Here's how the part is built. I have some questions about the finished solid (model axes, mm). Round coordinates to 2 decimals unless told otherwise and drop trailing zeros. Write each loop counter-clockwise with the first axis right and the second up, starting at its lowest first coordinate (ties: lowest second). Pieces come first, ordered by that corner, then holes. Notation, with made-up numbers: M 20,59 L 41,59 A15 cw 41,88 Z; hole C 55.5,-23 d4. An arc over 180 degrees is marked long. Use one line per item in the form item = value. Start each with the question number.
Q1. I'm going to push a flat-ended pin straight in: pin 1 Ø2.5 at (x, z) = (15.98, -0.88) entering from +Y. Where does the tip first touch, or does it pass through?
Q2. I want a section at B-B on x = 0.5. List the corners of the cut face in (y, z) for me (3 decimals).
Q3. I want a section at D-D on y = 1.5. List the corners of the cut face in (x, z) for me (3 decimals), and give its area (3 significant figures).
Q4. I want a section at A-A on z = 3.5. List the corners of the cut face in (x, y) for me.
Q5. I need wall thicknesses on line 1 along X through (y, z) = (1.75, -2); line 2 along X through (y, z) = (4.75, -0.25); line 3 along X through (y, z) = (3.75, 4). Which ranges of each line are inside material? Lowest first, please. Write a range as from..to.
Q6. We'd pull the mould along Z, two halves only. Please class faces 1 (the face through (20, 5, 0)), 2 (the face through (0, 9, 4.875)), 3 (the face through (-14.49, 5.42, -1.07)): +Z half, -Z half, draft (parallel to the pull), parting line (faces both ways), or undercut.
Q7. I want a section at C-C on z = -0.5. List the corners of the cut face in (x, y) for me.
```python
from build123d import *

# Parameters (mm, degrees)
SKETCH1_W           = 40
SKETCH1_H           = 9.75
SKETCH1_R           = 1.5
BOSS_EXTRUDE1_DEPTH = 11
CUT_EXTRUDE1_REACH  = 26.821


with BuildPart() as part:
    # Sketch1 → Boss-Extrude1 (new body)
    with BuildSketch(Plane(origin=(0, 0, 0), x_dir=(1, 0, 0), z_dir=(0, 1, 0))):
        Rectangle(SKETCH1_W, SKETCH1_H)
        with Locations(Location((-15.976056303, 0.875, 0), (0, 0, 270))):
            Circle(SKETCH1_R, mode=Mode.SUBTRACT)
        with Locations(Location((15.976056303, 0.875, 0), (0, 0, 90))):
            Circle(SKETCH1_R, mode=Mode.SUBTRACT)
    extrude(amount=BOSS_EXTRUDE1_DEPTH)

    # Sketch2 → Cut-Extrude1 (cut, up to next)
    with BuildSketch(Plane.XY.offset(4.875), mode=Mode.PRIVATE) as cut_extrude1_sk1:
        with BuildLine():
            ThreePointArc((3, 5.5), (2.121320344, 7.621320344), (0, 8.5))
            Line((0, 8.5), (0, 2.5))
            ThreePointArc((0, 2.5), (2.121320344, 3.378679656), (3, 5.5))
        make_face()
    cut_extrude1_tool1 = extrude(cut_extrude1_sk1.sketch, amount=-CUT_EXTRUDE1_REACH, mode=Mode.PRIVATE) & part.part
    # Sketch2 → Cut-Extrude1 (cut, up to next)
    with BuildSketch(Plane.XY.offset(4.875), mode=Mode.PRIVATE) as cut_extrude1_sk2:
        with BuildLine():
            Line((0, 2.5), (0, 8.5))
            ThreePointArc((0, 8.5), (-3, 5.5), (0, 2.5))
        make_face()
    cut_extrude1_tool2 = extrude(cut_extrude1_sk2.sketch, amount=-CUT_EXTRUDE1_REACH, mode=Mode.PRIVATE) & part.part
    # Sketch2 → Cut-Extrude1 (cut, up to next)
    with BuildSketch(Plane.XY.offset(4.875), mode=Mode.PRIVATE) as cut_extrude1_sk3:
        with BuildLine():
            ThreePointArc((3, 5.5), (2.121320344, 7.621320344), (0, 8.5))
            Line((0, 8.5), (0, 2.5))
            ThreePointArc((0, 2.5), (2.121320344, 3.378679656), (3, 5.5))
        make_face()
    cut_extrude1_tool3 = extrude(cut_extrude1_sk3.sketch, amount=-CUT_EXTRUDE1_REACH, mode=Mode.PRIVATE) & part.part
    # Sketch2 → Cut-Extrude1 (cut, up to next)
    with BuildSketch(Plane.XY.offset(4.875), mode=Mode.PRIVATE) as cut_extrude1_sk4:
        with BuildLine():
            Line((0, 2.5), (0, 8.5))
            ThreePointArc((0, 8.5), (-3, 5.5), (0, 2.5))
        make_face()
    cut_extrude1_tool4 = extrude(cut_extrude1_sk4.sketch, amount=-CUT_EXTRUDE1_REACH, mode=Mode.PRIVATE) & part.part
    add(cut_extrude1_tool1.solids().sort_by_distance((1.27324, 5.5, 4.875))[0], mode=Mode.SUBTRACT)
    add(cut_extrude1_tool2.solids().sort_by_distance((-1.27324, 5.5, 4.875))[0], mode=Mode.SUBTRACT)
    add(cut_extrude1_tool3.solids().sort_by_distance((1.27324, 5.5, 4.875))[0], mode=Mode.SUBTRACT)
    add(cut_extrude1_tool4.solids().sort_by_distance((-1.27324, 5.5, 4.875))[0], mode=Mode.SUBTRACT)


solid = part.part
```
Reported:
q1.pin_1 = through
q2.outline = M 0,-4.875 L 2.542,-4.875 L 2.542,4.875 L 0,4.875 Z; M 8.458,-4.875 L 11,-4.875 L 11,4.875 L 8.458,4.875 Z
q3.outline = M -20,-4.875 L 20,-4.875 L 20,4.875 L -20,4.875 Z; hole C -15.976,-0.875 d3; hole C 15.976,-0.875 d3
q3.area = 376 mm^2
q4.outline = M -20,0 L 20,0 L 20,11 L -20,11 Z; hole C 0,5.5 d6
q5.line_1 = -20..-16.97, -14.98..14.98, 16.97..20
q5.line_2 = -20..-17.34, -14.61..-2.9, 2.9..14.61, 17.34..20
q5.line_3 = -20..-2.44, 2.44..20
q6.face_1 = draft
q6.face_2 = +Z half
q6.face_3 = undercut
q7.outline = M -20,0 L -17.43,0 L -17.43,11 L -20,11 Z; M -14.52,0 L 14.52,0 L 14.52,11 L -14.52,11 Z; M 17.43,0 L 20,0 L 20,11 L 17.43,11 Z; hole C 0,5.5 d6
